Input: part model. Units: mm. Frame: model coordinates. A direction names the side the tool comes from. Coordinates: 2 decimals unless noted, no trailing zeros. Order: outer loops, then holes, each group sorted by start corner. A loop starts at its lowest first (then second) coordinate and runs counter-clockwise, first axis right, second up. Notation, with made-up numbers: M 17,1.5 L 76,1.5 A23 cw 76,27.5 Z; hole C 38.5,33 d6. An arc over 180 degrees is marked long. Answer in a Markdown table with one row per item.
from build123d import *

# Parameters (mm, degrees)
SKETCH_2_R          = 35
SKETCH_2_R_2        = 12
EXTRUDE_1_DEPTH     = 5
EXTRUDE_START       = 15
SKETCH_3_R          = 35
SKETCH_3_R_2        = 30.05
EXTRUDE_2_DEPTH     = 15
SKETCH_4_R          = 1.55
CUT_EXTRUDE_1_DEPTH = 10
FILLET_1_R          = 1
CUT_EXTRUDE_2_DEPTH = 52.720402193


with BuildPart() as part:
    # 草图2 → 凸台-拉伸1 (new body)
    with BuildSketch(Plane.XY):
        Circle(SKETCH_2_R)
        Circle(SKETCH_2_R_2, mode=Mode.SUBTRACT)
    extrude(amount=EXTRUDE_1_DEPTH)

    # 草图3 → 凸台-拉伸2 (add)
    with BuildSketch(Plane(origin=(0, 0, 0), x_dir=(-1, 0, 0), z_dir=(0, 0, -1)).offset(EXTRUDE_START)):
        Circle(SKETCH_3_R)
        Circle(SKETCH_3_R_2, mode=Mode.SUBTRACT)
    extrude(amount=-EXTRUDE_2_DEPTH)

    # 草图4 → 切除-拉伸1 (cut)
    with BuildSketch(Plane(origin=(0, 0, -15), x_dir=(-1, 0, 0), z_dir=(0, 0, -1))):
        with Locations((0, 32.5)):
            Circle(SKETCH_4_R)
        with Locations((32.5, 0)):
            Circle(SKETCH_4_R)
        with Locations((0, -32.5)):
            Circle(SKETCH_4_R)
        with Locations((-32.5, 0)):
            Circle(SKETCH_4_R)
    extrude(amount=-CUT_EXTRUDE_1_DEPTH, mode=Mode.SUBTRACT)

    # 圆角1
    # the kernel refuses this fillet: 1 mm, written as the material it takes off along each edge
    with BuildSketch(Plane(origin=(0, 0, -15), x_dir=(-1, 0, 0), z_dir=(0, -1, 0))) as fillet_1_piece_1:
        with BuildLine():
            CenterArc((30.05 + FILLET_1_R, -FILLET_1_R), FILLET_1_R, 90, 90)
            Line((30.05, -FILLET_1_R), (30.05, 0))
            Line((30.05, 0), (30.05 + FILLET_1_R, 0))
        make_face()
    revolve(axis=Axis((0, 0, -15), (0, 0, -1)), mode=Mode.SUBTRACT)

    # 草图5 → 切除-拉伸2 (cut, through all)
    with BuildSketch(Plane(origin=(0, 0, 0), x_dir=(-1, 0, 0), z_dir=(0, 0, -1))):
        with BuildLine():
            Line((12.990381057, -7.5), (15.588457268, -9))
            ThreePointArc((15.588457268, -9), (18, 0), (15.588457268, 9))
            Line((15.588457268, 9), (12.990381057, 7.5))
            ThreePointArc((12.990381057, 7.5), (15, 0), (12.990381057, -7.5))
        make_face()
        with BuildLine():
            Line((-7.5, 12.990381057), (-9, 15.588457268))
            ThreePointArc((-9, 15.588457268), (0, 18), (9, 15.588457268))
            Line((9, 15.588457268), (7.5, 12.990381057))
            ThreePointArc((7.5, 12.990381057), (0, 15), (-7.5, 12.990381057))
        make_face()
        with BuildLine():
            Line((-7.5, -12.990381057), (-9, -15.588457268))
            ThreePointArc((-9, -15.588457268), (0, -18), (9, -15.588457268))
            Line((9, -15.588457268), (7.5, -12.990381057))
            ThreePointArc((7.5, -12.990381057), (0, -15), (-7.5, -12.990381057))
        make_face()
        with BuildLine():
            Line((-12.990381057, 7.5), (-15.588457268, 9))
            ThreePointArc((-15.588457268, 9), (-18, 0), (-15.588457268, -9))
            Line((-15.588457268, -9), (-12.990381057, -7.5))
            ThreePointArc((-12.990381057, -7.5), (-15, 0), (-12.990381057, 7.5))
        make_face()
    extrude(amount=-CUT_EXTRUDE_2_DEPTH, mode=Mode.SUBTRACT)


solid = part.part
1) Cut plane D-D, the plane x = 14. State how many separate pieces and enclosed holes the cut face has, and give its area (3 significant figures).
Resolved:
| item | result |
|---|---|
| separate pieces | 3 |
| enclosed holes | 0 |
| area | 458 mm2 |
2) Contact query for flat-ended pins moving along their axis: pin 1 (8 mm diameter, centred on x = 19, z = -7.5, fed in from +Y); pin 2 (12 mm diameter, centred on x = -2.5, z = -5, fed in from +Y); pin 3 (12 mm diameter, centred on x = 22.5, z = -1.5, fed in from -Y). Output: stop coordinate, or through.
Resolved:
| item | result |
|---|---|
| pin 1 | stops at y = 31.62 |
| pin 2 | stops at y = 35 |
| pin 3 | stops at y = -30.87 |
3) Reachability of faces 3 (the face through (0, 15, 2)), 4 (the face through (0.202, 34.037, -10.07)) from +Z, -Z, +X, -X, +Y, -Y: full face, straight path, thin tool, end or side. Return the list, or none.
Resolved:
| item | result |
|---|---|
| face 3 | +Z, -Z |
| face 4 | -Z |
4) Mould query, pull axis X, two halves, no side actions, for faces 1 (the face through (-14.27, -8.24, 2.46)), 2 (the face through (20.9, -23.2, -15)). Classes: +X half, -X half, draft (parallel to the pull), parting line (faces both ways), or undercut.
Resolved:
| item | result |
|---|---|
| face 1 | undercut |
| face 2 | draft |
5) Cut plane A-A, the plane x = -32.5. Output: boundary loops of the cut face in (y, z).
Resolved:
| item | result |
|---|---|
| outline | M -12.99,-15 L -1.55,-15 L -1.55,-5 L 1.55,-5 L 1.55,-15 L 12.99,-15 L 12.99,5 L -12.99,5 Z |
6) Cut plane B-B, the plane z = 3. Output: boundary loops of the cut face in (x, y), and give its area (3 significant figures).
Resolved:
| item | result |
|---|---|
| outline | C 0,0 d70; hole M -15.59,-9 L -12.99,-7.5 A15 cw -12.99,7.5 L -15.59,9 A18 ccw Z; hole C 0,0 d24; hole M -9,-15.59 A18 ccw 9,-15.59 L 7.5,-12.99 A15 cw -7.5,-12.99 Z; hole M -9,15.59 L -7.5,12.99 A15 cw 7.5,12.99 L 9,15.59 A18 ccw Z; hole M 12.99,-7.5 L 15.59,-9 A18 ccw 15.59,9 L 12.99,7.5 A15 cw Z |
| area | 3,190 mm2 |
7) Material intervals for probe 1 along Y at (x, z) = (0, -11); probe 2 along Y at (x, z) = (0, -3.25); probe 3 along X at (y, z) = (-4, 1.75), sorted ascending.
Resolved:
| item | result |
|---|---|
| probe 1 | y = -35 to -34.05, -30.95 to -30.05, 30.05 to 30.95, 34.05 to 35 |
| probe 2 | y = -35 to -30.05, 30.05 to 35 |
| probe 3 | x = -34.77 to -17.55, -14.46 to -11.31, 11.31 to 14.46, 17.55 to 34.77 |
